Verification items for the finished model (mm, model axes). A direction names the side the tool comes from. Give positions to 0.01 mm unless a question says otherwise; leave off trailing zeros. Order: outer loops, then holes, each group sorted by start corner. A loop starts at its lowest first (then second) coordinate and runs counter-clockwise, first axis right, second up. Notation, with made-up numbers: M 38,59 L 90,59 A26 ccw 90,81 Z; hole C -26.5,48 d6. An arc over 180 degrees is marked long. Answer as a JSON object with one key per item and string values.
```python
from build123d import *

# Parameters (mm, degrees)
BOSS_EXTRUDE1_DEPTH = 6
FILLET1_R           = 0.5
SKETCH4_R           = 6
BOSS_EXTRUDE2_DEPTH = 6
SKETCH3_R           = 2
SKETCH3_R_2         = 6
CUT_EXTRUDE1_DEPTH  = 284.694910827
CUT_EXTRUDE2_REACH  = 285.695
SKETCH6_R           = 1.55


with BuildPart() as part:
    # Sketch2 → Boss-Extrude1 (new body)
    with BuildSketch(Plane(origin=(0, 0, 0), x_dir=(0, 0, -1), z_dir=(1, 0, 0))):
        Polygon((-30.67492643, 30.67492643), (-30.67492643, 257.67492643), (-5.67492643, 282.67492643), (-5.67492643, 5.67492643), align=None)
    extrude(amount=BOSS_EXTRUDE1_DEPTH)

    # Fillet1
    fillet1_edges = [part.edges().sort_by_distance(p)[0] for p in [
        (3, 282.67492643, 5.67492643),
        (3, 5.67492643, 5.67492643),
    ]]
    fillet(fillet1_edges, radius=FILLET1_R)

    # Sketch4 → Boss-Extrude2 (add)
    with BuildSketch(Plane(origin=(6, 0, 0), x_dir=(0, 0, -1), z_dir=(1, 0, 0))):
        with Locations((-17.67492643, 270.67492643)):
            Circle(SKETCH4_R)
    extrude(amount=-BOSS_EXTRUDE2_DEPTH)

    # Sketch3 → Cut-Extrude1 (cut, through all)
    with BuildSketch(Plane(origin=(6, 0, 0), x_dir=(0, 0, -1), z_dir=(1, 0, 0))):
        with Locations((-17.67492643, 270.67492643)):
            Circle(SKETCH3_R)
        with Locations((-17.67492643, 17.67492643)):
            Circle(SKETCH3_R_2)
    extrude(amount=-CUT_EXTRUDE1_DEPTH, mode=Mode.SUBTRACT)

    # Sketch6 → Cut-Extrude2 (cut, up to next)
    with BuildSketch(Plane(origin=(6, 0, 0), x_dir=(0, 0, -1), z_dir=(1, 0, 0)), mode=Mode.PRIVATE) as cut_extrude2_sk1:
        with Locations((-24.67492643, 94.17492643)):
            Circle(SKETCH6_R)
    cut_extrude2_tool1 = extrude(cut_extrude2_sk1.sketch, amount=-CUT_EXTRUDE2_REACH, mode=Mode.PRIVATE) & part.part
    # Sketch6 → Cut-Extrude2 (cut, up to next)
    with BuildSketch(Plane(origin=(6, 0, 0), x_dir=(0, 0, -1), z_dir=(1, 0, 0)), mode=Mode.PRIVATE) as cut_extrude2_sk2:
        with Locations((-24.67492643, 194.17492643)):
            Circle(SKETCH6_R)
    cut_extrude2_tool2 = extrude(cut_extrude2_sk2.sketch, amount=-CUT_EXTRUDE2_REACH, mode=Mode.PRIVATE) & part.part
    add(cut_extrude2_tool1.solids().sort_by_distance((6, 94.174926, 24.674926))[0], mode=Mode.SUBTRACT)
    add(cut_extrude2_tool2.solids().sort_by_distance((6, 194.174926, 24.674926))[0], mode=Mode.SUBTRACT)


solid = part.part
```
Q1. Material ranges on L1, parallel to Y at x = 4.65, z = 24.5; L2, parallel to Y at x = 0.7, z = 25; L3, parallel to Y at x = 2.35, z = 12.75, recorded low to high.
Resolved:
{"L1": "y = 24.5 to 92.63, 95.72 to 192.63, 195.72 to 263.85", "L2": "y = 25 to 92.66, 95.69 to 192.66, 195.69 to 263.35", "L3": "y = 12.75 to 14.25, 21.1 to 275.6"}
Q2. Tool access check on faces 1 (the face through (2.96, 261.99, 26.36)), 2 (the face through (3, 143, 30.675)). Record the directions out of +Z, -Z, +X, -X, +Y, -Y that give a thin tool (end or side, any length) a straight path to the whole face; none if there is none.
Resolved:
{"face 1": "+Z, +X, -X", "face 2": "+Z, +X, -X, +Y, -Y"}
Q3. Release check for a two-part mould opening along Z. For faces 3 (the face through (0, 146, 18)), 4 (the face through (3, 10, 10)), 5 (the face through (2.96, 278.32, 10.03)) record: +Z half, -Z half, draft (parallel to the pull), parting line (faces both ways), or undercut.
Resolved:
{"face 3": "draft", "face 4": "+Z half", "face 5": "undercut"}
Q4. Section check A-A on x = 3.45. Record the cut outline in (y, z).
Resolved:
{"outline": "M 6.53,6.53 A0.5 ccw 6.88,5.67 L 281.47,5.67 A0.5 ccw 281.82,6.53 L 274.92,13.43 A6 ccw 266.43,21.92 L 257.67,30.67 L 30.67,30.67 L 21.92,21.92 A6 cw 13.43,13.43 Z; hole C 94.17,24.67 d3.1; hole C 194.17,24.67 d3.1; hole C 270.67,17.67 d4"}
